Build history of the part. All positions in model axes, mm. A direction names the side the tool comes from. Give positions to 0.01 mm unless a question says otherwise; leave off trailing zeros. Use a Markdown table: item, result.
from build123d import *

# Parameters (mm, degrees)
F0_R     = 127
F1_DEPTH = 25.4
F2_R     = 120.65
F2_R_2   = 115.57
F4_DEPTH = 6.35
F3_R     = 22.225
F6_DEPTH = 15.24
F7_D     = 12.7
F7_DEPTH = 12.7
F7_TIP   = 3.8154649308
F8_R     = 1.27
F9_SIZE  = 1.27


with BuildPart() as f1:
    # F0 (on Top) → F1 (new body)
    with BuildSketch(Plane.XY):
        Circle(F0_R)
    extrude(amount=F1_DEPTH)

    # F2 (on face) → F4 (cut)
    with BuildSketch(Plane(origin=(0, 0, 0), x_dir=(1, 0, 0), z_dir=(0, 0, -1))):
        Circle(F2_R)
        Circle(F2_R_2, mode=Mode.SUBTRACT)
    extrude(amount=-F4_DEPTH, mode=Mode.SUBTRACT)

    # F3 (on Top) → F6 (cut)
    with BuildSketch(Plane.XY):
        Circle(F3_R)
    extrude(amount=F6_DEPTH, mode=Mode.SUBTRACT)

    # F7
    with Locations(Plane(origin=(0, 0, 0), x_dir=(1, 0, 0), z_dir=(0, 0, -1))):
        with Locations((31.75, 0), (-31.75, 0)):
            Hole(F7_D / 2, depth=F7_DEPTH)
            with Locations((0, 0, -(F7_DEPTH + F7_TIP / 2))):  # 118° drill point
                Cone(0, F7_D / 2, F7_TIP, mode=Mode.SUBTRACT)

    # F8
    f8_edges = [f1.edges().sort_by_distance(p)[0] for p in [
        (-22.225, 0, 15.24),
        (-127, 0, 25.4),
    ]]
    fillet(f8_edges, radius=F8_R)

    # F9
    f9_edges = [f1.edges().sort_by_distance(p)[0] for p in [
        (-22.225, 0, 0),
        (-115.57, 0, 0),
        (-120.65, 0, 0),
        (-127, 0, 0),
        (-38.1, 0, 0),
        (25.4, 0, 0),
    ]]
    chamfer(f9_edges, length=F9_SIZE)


solid = f1.part
1) Wall check: line 1 (Y direction, x = 0, z = 4.35) (3 decimals); line 2 (Y direction, x = 0, z = 8.5) (3 decimals); line 3 (Y direction, x = -10.5, z = 2). Give the ranges that are in metal, low to high. Write a range as from..to.
Computed:
| item | result |
|---|---|
| line 1 | y = -127..-120.65, -115.57..-22.225, 22.225..115.57, 120.65..127 |
| line 2 | y = -127..-22.225, 22.225..127 |
| line 3 | y = -126.57..-120.19, -115.09..-19.59, 19.59..115.09, 120.19..126.57 |
2) Tool access for faces 4 (the cylindrical face through (25.693, -1.907, 7.065)), 5 (the flat face through (-2, 2, 25.4)): list every direction of +Z, -Z, +X, -X, +Y, -Y with a clear straight run to the whole face (end or side of a thin tool).
Computed:
| item | result |
|---|---|
| face 4 | -Z |
| face 5 | +Z, +X, -X, +Y, -Y |
3) Pin check, flat tips, straight feed: P1, Ø5, axis at x = -51.5, z = 14.5, coming from the -Y side; P2, Ø5, axis at x = 12, z = 10.5, coming from the -Y side; P3, Ø10, axis at x = 49.5, z = 9.5, coming from the -Y side. Stop position of each tip, or through.
Computed:
| item | result |
|---|---|
| P1 | stops at y = -117.17 |
| P2 | stops at y = -126.64 |
| P3 | stops at y = -118.95 |
4) Two-plate mould, pull along Y, no slides. Class faces 1 (the conical face through (32.802, -0.331, 15.853)), 2 (the cylindrical face through (-27.53, -123.98, 12.54)), 3 (the flat face through (-103, 66, 0)): +Y half, -Y half, draft (parallel to the pull), parting line (faces both ways), or undercut.
Computed:
| item | result |
|---|---|
| face 1 | undercut |
| face 2 | parting line |
| face 3 | draft |
